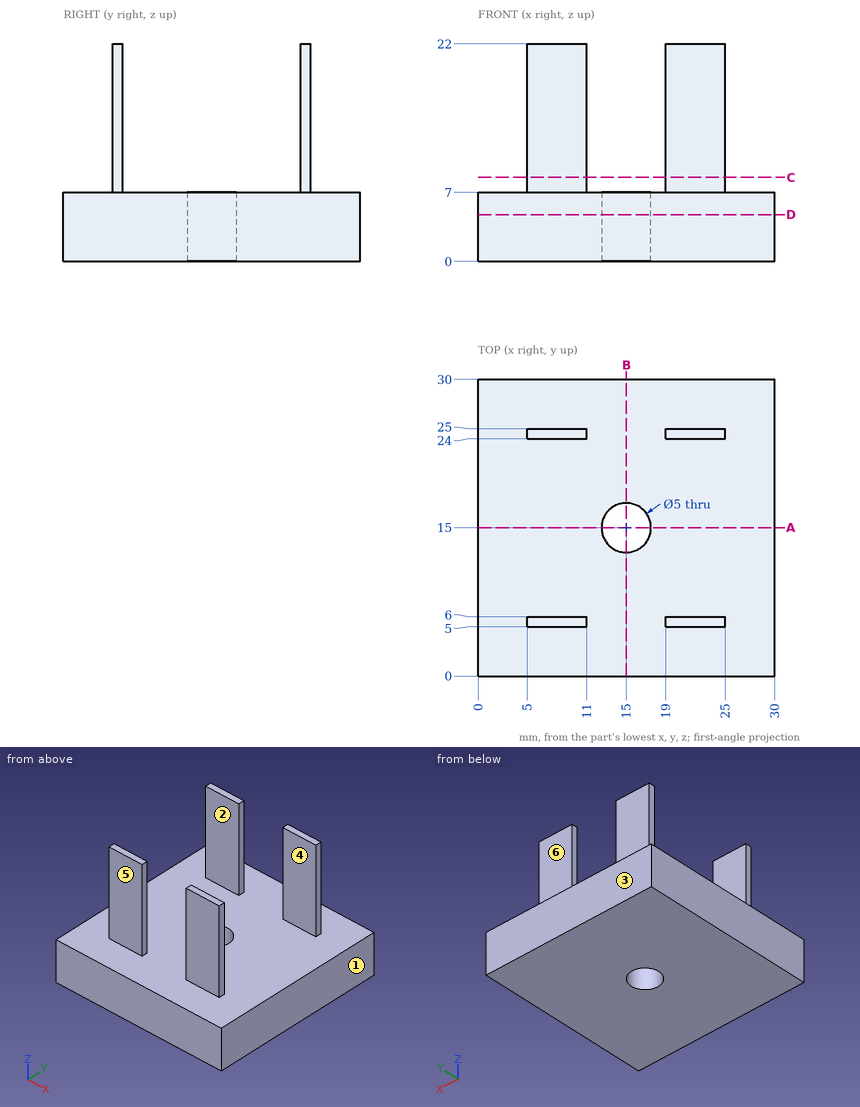
For this review, use the dimensioned drawing (mm, ordinates from the lowest corner) and the shaded views. A direction names the side the tool comes from. Coordinates: 2 decimals unless noted, no trailing zeros. Order: outer loops, then holes, each group sorted by start corner. A loop starts at its lowest first (then second) coordinate and runs counter-clockwise, first axis right, second up. Notation, with made-up numbers: (74.25, 59.25) - (132.25, 59.25) arc R21 cw to (132.25, 66.25) - close; hole circle Ø9 at (-6, 44). An arc over 180 degrees is marked (long way). Answer in a Markdown table with one row per item.
(1) Consider section D-D on z = 4.75. State the section outline as (x, y) points, plus the area to 3 significant figures.
Checked values:
| item | result |
|---|---|
| outline | (0, 0) - (30, 0) - (30, 30) - (0, 30) - close; hole circle Ø5 at (15, 15) |
| area | 880 mm^2 |
(2) Clearance check with flat-ended pins moving along their axes: pin 1 (3 mm diameter, centred on x = 20.5, z = 12.5, fed in from -Y); pin 2 (1.5 mm diameter, centred on x = 10.5, y = 5, fed in from -Z); pin 3 (0.8 mm diameter, centred on y = 5.5, z = 16, fed in from -X); pin 4 (8 mm diameter, centred on x = 5.5, z = 13.5, fed in from +Y). State where each tip first meets the part, or that it passes through.
Checked values:
| item | result |
|---|---|
| pin 1 | y = 5 |
| pin 2 | z = 0 |
| pin 3 | x = 5 |
| pin 4 | y = 25 |
(3) Wall thickness on line 1 along Y through (x, z) = (5.5, 20.25); line 2 along Y through (x, z) = (15, 4); line 3 along Z through (x, y) = (19.25, 27): over which ranges is each line inside the solid? List them lowest first. Write a range as from..to.
Checked values:
| item | result |
|---|---|
| line 1 | 5..6, 24..25 |
| line 2 | 0..12.5, 17.5..30 |
| line 3 | 0..7 |
(4) For the marked faces 4, 5 and 6, list the 3-axis set-ups (+Z, -Z, +X, -X, +Y, -Y) from which the entire face can be reached by the end or side of a thin tool; tool diameter is ignored.
Checked values:
| item | result |
|---|---|
| face 4 | +Z, +X, -X |
| face 5 | +Z, +X, -X, -Y |
| face 6 | +Z, +X, -X, +Y |
(5) The part is to be moulded in two halves that separate along Y. For the marked faces 1, 2 and 3, say which applies: released by +Y, released by -Y, zero draft, split by the parting line, or undercut.
Checked values:
| item | result |
|---|---|
| face 1 | zero draft |
| face 2 | undercut |
| face 3 | released by +Y |
(6) Consider section A-A on y = 15. State the section outline as (x, z) points, plus the area to 3 significant figures.
Checked values:
| item | result |
|---|---|
| outline | (0, 0) - (12.5, 0) - (12.5, 7) - (0, 7) - close; (17.5, 0) - (30, 0) - (30, 7) - (17.5, 7) - close |
| area | 175 mm^2 |
(7) Consider section C-C on z = 8.5. State the section outline as (x, y) points, plus the area to 3 significant figures.
Checked values:
| item | result |
|---|---|
| outline | (5, 5) - (11, 5) - (11, 6) - (5, 6) - close; (5, 24) - (11, 24) - (11, 25) - (5, 25) - close; (19, 5) - (25, 5) - (25, 6) - (19, 6) - close; (19, 24) - (25, 24) - (25, 25) - (19, 25) - close |
| area | 24.0 mm^2 |
